Geometry check sheet. Reference: the model listing, model coordinates, mm. Give positions to 0.01 mm unless a question says otherwise; leave off trailing zeros. Write each loop counter-clockwise with the first axis right and the second up, starting at its lowest first coordinate (ties: lowest second). Pieces come first, ordered by that corner, then holes. Notation, with made-up numbers: (-32.75, -5.5) - (-9.75, -5.5) arc R29 cw to (-9.75, 32.5) - close; hole circle Ø11 at (-20, 61.5). An arc over 180 degrees is marked (long way). Write item = value, one per line. Start each with the question number.
(1) Thickness scan on L1, parallel to X at y = 8, z = -17.5; L2, parallel to X at y = 6.75, z = -16; L3, parallel to X at y = 4.75, z = -31. Record the ranges inside material, lowest first.
(2) Section check A-A, the plane y = 9. Enter the section's corners in (x, z), plus the area to 3 significant figures.
(3) Section check D-D, the plane x = 32. Enter the section's corners in (y, z), plus the area to 3 significant figures.
(4) Section check C-C, the plane x = 17.5. Enter the section's corners in (y, z).
(5) Depth check by flat-ended pin: pin 1 Ø1.5 at (y, z) = (10.5, -30) entering from -X; pin 2 Ø4 at (x, z) = (17.5, -17.5) entering from -Y. Enter the tip coordinate at first touch or a pass-through.
(6) Draft check along Z on faces 1 (the cylindrical face through (17.6, 6.3, -20)), 2 (the flat face through (32.3, 6.3, -2.6)), 3 (the flat face through (17, 0, -14)). Enter one of: pulls with the +Z half, pulls with the -Z half, needs draft (parallel to the pull), parting line crosses it, or undercut.
(7) Section check B-B, the plane z = -17.5. Enter the section's corners in (x, y), plus the area to 3 significant figures.
```python
from build123d import *

# Parameters (mm, degrees)
CROQUIS1_W              = 35
CROQUIS1_H              = 35
SALIENTE_EXTRUIR1_DEPTH = 12.4
CROQUIS2_OUTSIDE_W      = 47.206
CROQUIS2_OUTSIDE_H      = 47.206
CORTAR_EXTRUIR2_DEPTH   = 18
CROQUIS3_R              = 2.5
CORTAR_EXTRUIR3_DEPTH   = 52.027051649


with BuildPart() as part:
    # Croquis1 → Saliente-Extruir1 (new body)
    with BuildSketch(Plane(origin=(0, 0, 0), x_dir=(1, 0, 0), z_dir=(0, 1, 0))):
        with Locations((17.5, 17.5)):
            Rectangle(CROQUIS1_W, CROQUIS1_H)
    extrude(amount=SALIENTE_EXTRUIR1_DEPTH)

    # Croquis2 outside → Cortar-Extruir2 (cut)
    with BuildSketch(Plane(origin=(0, 12.4, 0), x_dir=(1, 0, 0), z_dir=(0, 1, 0))):
        with Locations((17.5, 17.5)):
            Rectangle(CROQUIS2_OUTSIDE_W, CROQUIS2_OUTSIDE_H)
        Polygon((5.30151519, 35), (0, 29.69848481), (0, 5.30151519), (5.30151519, 0), (29.69848481, 0), (35, 5.30151519), (35, 29.69848481), (29.69848481, 35), align=None, mode=Mode.SUBTRACT)
    extrude(amount=-CORTAR_EXTRUIR2_DEPTH, mode=Mode.SUBTRACT)

    # Croquis3 → Cortar-Extruir3 (cut, through all)
    with BuildSketch(Plane(origin=(0, 12.4, 0), x_dir=(1, 0, 0), z_dir=(0, 1, 0))):
        with Locations(Location((17.5, 17.5, 0), (0, 0, 270))):
            Circle(CROQUIS3_R)
    extrude(amount=-CORTAR_EXTRUIR3_DEPTH, mode=Mode.SUBTRACT)


solid = part.part
```
Model answer:
q1.L1 = 0 to 15, 20 to 35
q1.L2 = 0 to 15.5, 19.5 to 35
q1.L3 = 1.3 to 33.7
q2.outline = (0, -29.7) - (5.3, -35) - (29.7, -35) - (35, -29.7) - (35, -5.3) - (29.7, 0) - (5.3, 0) - (0, -5.3) - close; hole circle Ø5 at (17.5, -17.5)
q2.area = 1,150 mm²
q3.outline = (0, -32.7) - (12.4, -32.7) - (12.4, -2.3) - (0, -2.3) - close
q3.area = 377 mm²
q4.outline = (0, -35) - (12.4, -35) - (12.4, -20) - (0, -20) - close; (0, -15) - (12.4, -15) - (12.4, 0) - (0, 0) - close
q5.pin_1 = 0
q5.pin_2 = through
q6.face_1 = undercut
q6.face_2 = pulls with the +Z half
q6.face_3 = needs draft
q7.outline = (0, 0) - (15, 0) - (15, 12.4) - (0, 12.4) - close; (20, 0) - (35, 0) - (35, 12.4) - (20, 12.4) - close
q7.area = 372 mm²
